Geometry: see drawing. Coordinates: mm, zero at the bounding-box minimum. A direction names the side the tool comes from. Give positions to 0.01 mm unless a question says otherwise; leave off trailing zeros. Order: outer loops, then holes, each group sorted by start corner. A loop starts at its lowest first (then second) coordinate and runs counter-clockwise, first axis right, second up. Notation, with made-up numbers: M 61.5,72 L 65.5,72 A20 cw 65.5,87 Z; hole C -25.75,36.5 d6. An arc over 180 degrees is marked long. Use a Markdown table: item, result.
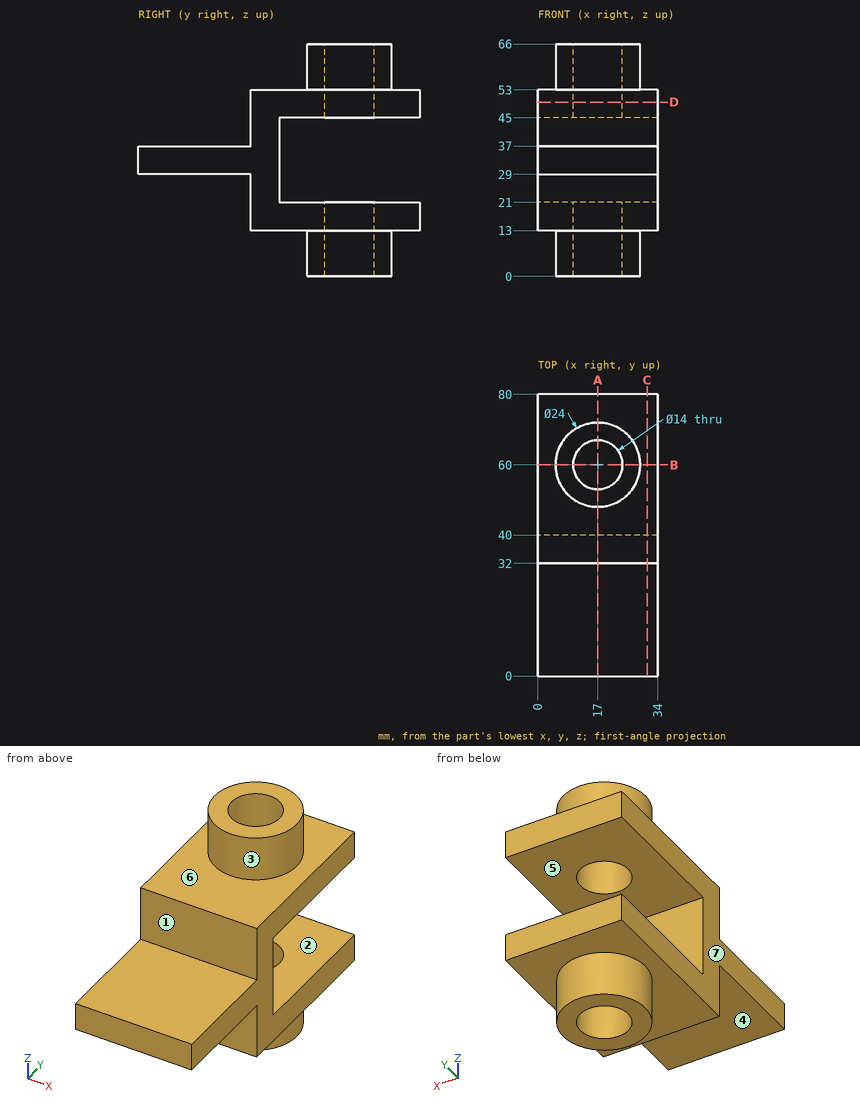
1) Mould query, pull axis Z, two halves, no side actions, for the marked faces 5, 6 and 7. Classes: released by +Z, released by -Z, zero draft, split by the parting line, or undercut.
Response values:
| item | result |
|---|---|
| face 5 | undercut |
| face 6 | released by +Z |
| face 7 | zero draft |
2) Cut plane C-C on x = 31. Return loops of the section in (y, z).
Response values:
| item | result |
|---|---|
| outline | M 0,29 L 32,29 L 32,13 L 80,13 L 80,21 L 40,21 L 40,45 L 80,45 L 80,53 L 32,53 L 32,37 L 0,37 Z |
3) Cut plane B-B on y = 60. Return loops of the section in (x, z).
Response values:
| item | result |
|---|---|
| outline | M 0,13 L 5,13 L 5,0 L 10,0 L 10,21 L 0,21 Z; M 0,45 L 10,45 L 10,66 L 5,66 L 5,53 L 0,53 Z; M 24,0 L 29,0 L 29,13 L 34,13 L 34,21 L 24,21 Z; M 24,45 L 34,45 L 34,53 L 29,53 L 29,66 L 24,66 Z |
4) Reachability of the marked faces 1, 2, 3 and 4 from +Z, -Z, +X, -X, +Y, -Y: full face, straight path, thin tool, end or side. Return the list, or none.
Response values:
| item | result |
|---|---|
| face 1 | +Z, +X, -X, -Y |
| face 2 | +X, -X, +Y |
| face 3 | +Z |
| face 4 | -Z, +X, -X, -Y |
5) Cut plane D-D on z = 49.5. Return loops of the section in (x, y).
Response values:
| item | result |
|---|---|
| outline | M 0,32 L 34,32 L 34,80 L 0,80 Z; hole C 17,60 d14 |
6) First-contact query: pin 1 Ø8.5 at (x, y) = (17, 60) entering from +Z; pin 2 Ø16 at (x, y) = (16.5, 11) entering from -Z; pin 3 Ø3 at (x, z) = (22, 51) entering from -Y; pin 4 Ø8 at (x, z) = (13, 36.5) entering from +Y. Flat tips, straight axial feed; report the tip coordinate or a pass-through.
Response values:
| item | result |
|---|---|
| pin 1 | passes through |
| pin 2 | stops at z = 29 |
| pin 3 | stops at y = 32 |
| pin 4 | stops at y = 40 |
7) Material intervals for line 1 (Y direction, x = 17, z = 16.75); line 2 (Y direction, x = 17, z = 57); line 3 (Z direction, x = 31, y = 43), sorted ascending. Write a range as from..to.
Response values:
| item | result |
|---|---|
| line 1 | y = 32..53, 67..80 |
| line 2 | y = 48..53, 67..72 |
| line 3 | z = 13..21, 45..53 |
8) Cut plane A-A on x = 17. Return loops of the section in (y, z).
Response values:
| item | result |
|---|---|
| outline | M 0,29 L 32,29 L 32,13 L 48,13 L 48,0 L 53,0 L 53,21 L 40,21 L 40,45 L 53,45 L 53,66 L 48,66 L 48,53 L 32,53 L 32,37 L 0,37 Z; M 67,0 L 72,0 L 72,13 L 80,13 L 80,21 L 67,21 Z; M 67,45 L 80,45 L 80,53 L 72,53 L 72,66 L 67,66 Z |
